```python
from build123d import *

# Parameters (mm, degrees)
SKETCH_W        = 50
SKETCH_H        = 85
PAD_DEPTH       = 50
POCKET_DEPTH    = 50
POCKET001_DEPTH = 30
SKETCH003_W     = 16
SKETCH003_H     = 26
POCKET002_DEPTH = 26
SKETCH004_R     = 2
POCKET003_DEPTH = 4
SKETCH005_R     = 2
POCKET004_DEPTH = 4
POCKET005_DEPTH = 2
SKETCH007_W     = 44
SKETCH007_H     = 60
POCKET006_DEPTH = 32
SKETCH008_R     = 12.5
SKETCH008_R_2   = 1.5
SKETCH008_R_3   = 5.95
POCKET007_DEPTH = 18
SKETCH009_W     = 44
SKETCH009_H     = 60
POCKET008_DEPTH = 8
POCKET009_DEPTH = 50.001
FILLET_R        = 1


with BuildPart() as part:
    # Sketch → Pad (new body)
    with BuildSketch(Plane.YZ):
        Rectangle(SKETCH_W, SKETCH_H)
    extrude(amount=PAD_DEPTH)

    # Sketch001 (on Face6 of Pad) → Pocket (cut)
    with BuildSketch(Plane.YZ.offset(50)):
        Polygon((-25, -22.5), (-25, -42.5), (-5, -42.5), (-5, -22.5), (-12.51604, -22.5), (-12.51604, -24.5), (-9.81604, -24.5), (-13, -27.68), (-17, -27.68), (-20.18396, -24.5), (-17.48396, -24.5), (-17.48396, -22.5), align=None)
    extrude(amount=-POCKET_DEPTH, mode=Mode.SUBTRACT)

    # Sketch002 (on Face3 of Pocket) → Pocket001 (cut)
    with BuildSketch(Plane.ZX.offset(25)):
        Polygon((-22.5, 50), (-42.5, 50), (-42.5, 30), (-22.5, 30), (-22.5, 37.52), (-24.5, 37.52), (-24.5, 34.82), (-27.68, 38), (-27.68, 42), (-24.5, 45.18), (-24.5, 42.48), (-22.5, 42.48), align=None)
    extrude(amount=-POCKET001_DEPTH, mode=Mode.SUBTRACT)

    # Sketch003 (on Face3 of Pocket001) → Pocket002 (cut)
    with BuildSketch(Plane.ZX.offset(25)):
        with Locations((-32.5, 13)):
            Rectangle(SKETCH003_W, SKETCH003_H)
    extrude(amount=-POCKET002_DEPTH, mode=Mode.SUBTRACT)

    # Sketch004 (on Face30 of Pocket002) → Pocket003 (cut)
    with BuildSketch(Plane.ZX.offset(-1)):
        with Locations((-32.5, 13)):
            Circle(SKETCH004_R)
    extrude(amount=-POCKET003_DEPTH, mode=Mode.SUBTRACT)

    # Sketch005 (on Face8 of Pocket003) → Pocket004 (cut)
    with BuildSketch(Plane(origin=(26, 0, 0), x_dir=(0, 1, 0), z_dir=(-1, 0, 0))):
        with Locations((12, 32.5)):
            Circle(SKETCH005_R)
    extrude(amount=-POCKET004_DEPTH, mode=Mode.SUBTRACT)

    # Sketch006 (on Face10 of Pocket004) → Pocket005 (cut)
    with BuildSketch(Plane.YX.offset(42.5)):
        Polygon((-1, 0), (25, 26), (25, 0), align=None)
    extrude(amount=-POCKET005_DEPTH, mode=Mode.SUBTRACT)

    # Sketch007 (on Face5 of Pocket005) → Pocket006 (cut)
    with BuildSketch(Plane.YZ.offset(50)):
        with Locations((0, 12.5)):
            Rectangle(SKETCH007_W, SKETCH007_H)
    extrude(amount=-POCKET006_DEPTH, mode=Mode.SUBTRACT)

    # Sketch008 (on Face6 of Pocket006) → Pocket007 (cut)
    with BuildSketch(Plane.YZ.offset(18)):
        with Locations((0, 3.5)):
            Circle(SKETCH008_R)
        with Locations((-15, 18.5)):
            Circle(SKETCH008_R_2)
        with Locations((15, 18.5)):
            Circle(SKETCH008_R_2)
        with Locations((15, -11.5)):
            Circle(SKETCH008_R_2)
        with Locations((-15, -11.5)):
            Circle(SKETCH008_R_2)
        with Locations((0, 25.5)):
            Circle(SKETCH008_R_3)
    extrude(amount=-POCKET007_DEPTH, mode=Mode.SUBTRACT)

    # Sketch009 (on Face2 of Pocket007) → Pocket008 (cut)
    with BuildSketch(Plane(origin=(0, 0, 0), x_dir=(0, 1, 0), z_dir=(-1, 0, 0))):
        with Locations((0, -12.5)):
            Rectangle(SKETCH009_W, SKETCH009_H)
    extrude(amount=-POCKET008_DEPTH, mode=Mode.SUBTRACT)

    # Sketch010 (on Face11 of Pocket008) → Pocket009 (cut, through all)
    with BuildSketch(Plane(origin=(0, -25, 0), x_dir=(0, 0, -1), z_dir=(0, -1, 0))):
        Polygon((17.5, 50), (-42.5, 50), (-42.5, 25), align=None)
    extrude(amount=-POCKET009_DEPTH, mode=Mode.SUBTRACT)

    # Fillet
    fillet_edges = [part.edges().sort_by_distance(p)[0] for p in [
        (18, 0, 42.5),
        (0, -23.5, 42.5),
        (4, -22, 42.5),
        (8, 0, 42.5),
        (4, 22, 42.5),
        (0, 23.5, 42.5),
        (12.5, 25, 42.5),
        (25, 23.5, 42.5),
        (21.5, 22, 42.5),
        (21.5, -22, 42.5),
        (25, -23.5, 42.5),
        (12.5, -25, 42.5),
    ]]
    fillet(fillet_edges, radius=FILLET_R)


solid = part.part
```
Can you work these out from the model? Positions are in its coordinate system, mm. A direction names the side the tool comes from. Coordinates: 2 decimals unless noted, no trailing zeros. Loops run counter-clockwise (first coordinate to the right, second up) from the corner with the lowest first, then second, coordinate; pieces in that order, holes last. Notation, with made-up numbers: (85.25, 3) -> (119.25, 3) arc R24 ccw to (119.25, 31) -> close; hole circle Ø6 at (79, -11). An arc over 180 degrees is marked (long way). Put each result on its own line as item: value. Start each with the question number.
Q1. Thinking about a two-plate mould opening in Z: for faces 1 (the face through (13.07, 13.89, 19.51)), 2 (the face through (13, -2, 42.5)), 3 (the face through (25.35, -18.57, -26.11)), which applies, pulls with the +Z half, pulls with the -Z half, needs draft (parallel to the pull), parting line crosses it, or undercut?
Q2. I want a section at C-C (z = -32.5). Write out the boundary of the cut face in (x, y), plus the area to 3 significant figures.
Q3. For faces 4 (the face through (4, -22, 12)), 5 (the face through (25, -17.484, -24)), 6 (the face through (34, 0, -17.5)), 7 (the face through (25.35, -11.39, -26.07)), which set-ups out of +Z, -Z, +X, -X, +Y, -Y let a thin tool reach every point of the face, with its end or its side?
Q4. I want a section at D-D (z = 3.5). Write out the boundary of the cut face in (x, y), plus the area to 4 significant figures.
Q5. If I drill on line 1 (Z direction, x = 15, y = 15); line 2 (Z direction, x = 11, y = -15); line 3 (X direction, y = -2.65, z = -32.5), over which ranges is the centre line in solid material (lowest first)? Write a range as [from, to].
Q6. I'm going to push flat-ended pins straight in: P1, Ø8, axis at y = -7.5, z = 32, coming from the -X side; P2, Ø3.5, axis at y = 15, z = 18.5, coming from the +X side; P3, Ø2, axis at x = 38.5, y = -4.5, coming from the +Z side; P4, Ø3, axis at x = 37.5, z = 15.5, coming from the +Y side. Where does each tip first touch, or does it pass through?
Q7. I want a section at A-A (y = 0). Count the separate pieces of the cut face and the enclosed holes in it, plus the area to 3 significant figures.
Taken from the geometry:
1. face 1: undercut
1. face 2: pulls with the +Z half
1. face 3: pulls with the -Z half
2. outline: (0, -5) -> (11, -5) -> (11, -1) -> (0, -1) -> close; (15, -5) -> (30, -5) -> (30, 10) -> (26, 10) -> (26, -1) -> (15, -1) -> close; (26, 14) -> (30, 14) -> (30, 25) -> (26, 25) -> close
2. area: 192 mm2
3. face 4: +Z, -X
3. face 5: +X, -X, -Y
3. face 6: +Z, +X
3. face 7: -Z, +X, -X
4. outline: (0, -25) -> (41.25, -25) -> (41.25, -22) -> (18, -22) -> (18, -12.5) -> (8, -12.5) -> (8, -22) -> (0, -22) -> close; (0, 22) -> (8, 22) -> (8, 12.5) -> (18, 12.5) -> (18, 22) -> (41.25, 22) -> (41.25, 25) -> (0, 25) -> close
4. area: 437.5 mm2
5. line 1: z = [-24.5, -13], [-10, 17], [20, 42.5]
5. line 2: z = [-27.68, -13], [-10, 17], [20, 42.5]
5. line 3: x = [0, 11], [15, 30]
6. P1: stops at x = 8
6. P2: stops at x = 18
6. P3: stops at z = -17.5
6. P4: stops at y = 25
7. separate pieces: 3
7. enclosed holes: 0
7. area: 695 mm2
